Autodesk Inventor part; units mm, degrees
ref_plane "YZ Plane" through (0, 0, 0) normal (1, 0, 0) x (0, 1, 0)
ref_plane "XZ Plane" through (0, 0, 0) normal (0, 1, 0) x (-1, 0, 0)
ref_plane "XY Plane" through (0, 0, 0) normal (0, 0, 1) x (1, 0, 0)
sketch "Sketch4" plane through (0, 0, 0) normal (0, 1, 0) x (-1, 0, 0)
  line L0 (0, 0) -> (0, -1500)
  line L1 (550, -950) -> (550, -550)
  line L2 (150, -150) -> (150, -230)
  line L3 (150, -230) -> (230, -230)
  line L4 (550, -550) -> (230, -230)
  line L5 (150, -150) -> (0, 0)
  line L6 (150, -1350) -> (150, -1270)
  line L7 (150, -1270) -> (230, -1270)
  line L8 (0, -1500) -> (150, -1350)
  line L9 (230, -1270) -> (550, -950)
  dimension "d8" = 1500
  dimension "d11" = 550
  dimension "d12" = 80
  dimension "d13" = 150
  dimension "d14" = 150
  dimension "d15" = 80
  dimension "d16" = 45
extrude "Extrusion1" add sketch "Sketch4" along normal blind 20
fillet "Fillet1" radius 5 1 edges at (-150, 10, -230)
fillet "Fillet2" radius 5 1 edges at (-150, 10, -1270)
properties part number "top long"
Check sheet for the modelled part. Datum: model origin and axes. Units: mm. Round coordinates to 2 decimals unless told otherwise and drop trailing zeros. Loops run counter-clockwise (first coordinate to the right, second up) from the corner with the lowest first, then second, coordinate; pieces in that order, holes last. Notation, with made-up numbers: M -9,-32 L 41,-32 A17 cw 41,-15 Z; hole C 70,68 d8. An arc over 180 degrees is marked long. One line per question, with ' | ' between items. Start each with the question number.
Item 1: Section check B-B (x = -395). Record the boundary of the cut face in (y, z).
Item 2: Scan lines: probe 1 along Z at (x, y) = (-174, 1.5); probe 2 along Z at (x, y) = (-391.5, 8.75); probe 3 along X at (y, z) = (11, -332). Record each from-to range of solid material in increasing order.
Item 3: Section check A-A (y = 17). Record the boundary of the cut face in (x, z), and give its area (3 significant figures).
Item 4: Gauge pin test, flat ends, axial feed: pin 1 Ø6 at (x, y) = (-193.5, 6.5) entering from -Z; pin 2 Ø10 at (x, y) = (-389.5, 4.5) entering from -Z; pin 3 Ø3 at (x, y) = (-62.5, 9.5) entering from -Z. Record the tip position at first contact, or that the pin passes through.
Item 5: Section check C-C (z = -202.5). Record the boundary of the cut face in (x, y).
Worked out:
1) outline: M 0,-1105 L 20,-1105 L 20,-395 L 0,-395 Z
2) probe 1: -1270 to -230 | probe 2: -1108.5 to -391.5 | probe 3: -332 to 0
3) outline: M -550,-950 L -230,-1270 L -155,-1270 A5 cw -150,-1275 L -150,-1350 L 0,-1500 L 0,0 L -150,-150 L -150,-225 A5 cw -155,-230 L -230,-230 L -550,-550 Z | area: 516,000 mm^2
4) pin 1: z = -1270 | pin 2: z = -1115.5 | pin 3: z = -1439
5) outline: M -150,0 L 0,0 L 0,20 L -150,20 Z
